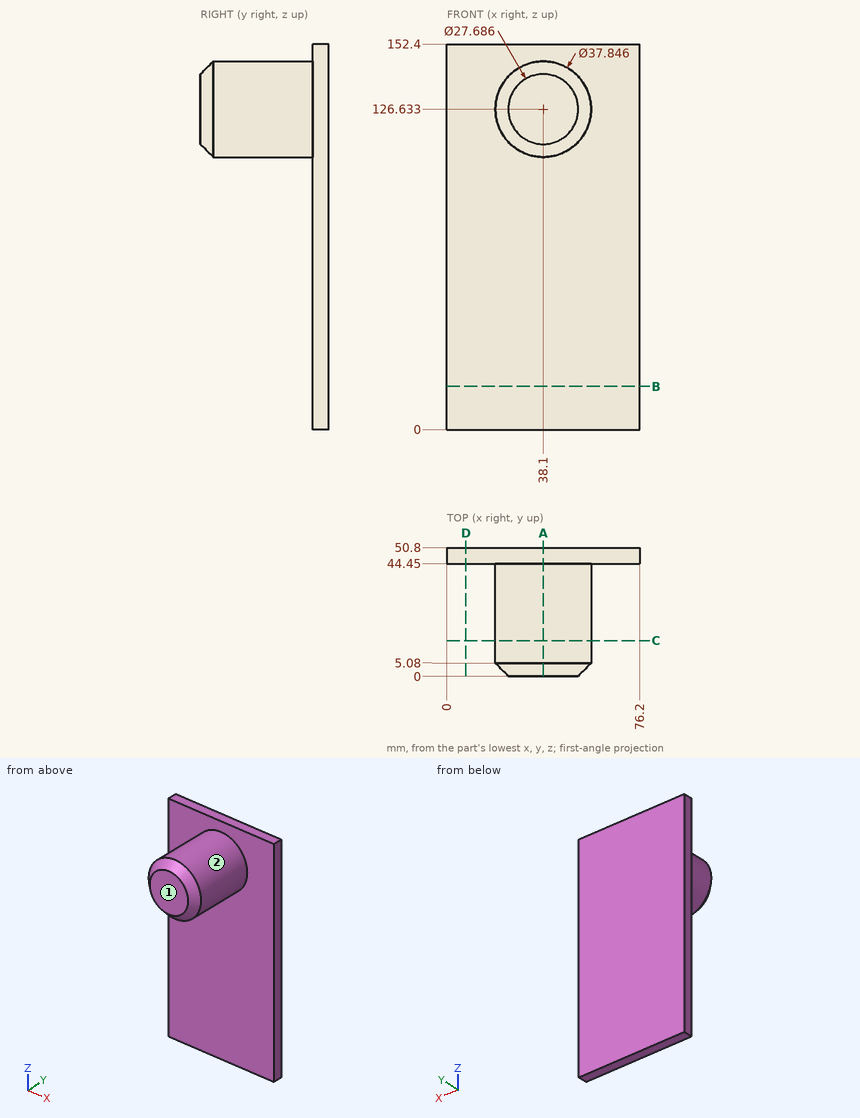
Here's the drawing with two shaded views (mm, measured from the low corner). I have some questions. A direction names the side the tool comes from. Give positions to 0.01 mm unless a question says otherwise; leave off trailing zeros. Order: outer loops, then holes, each group sorted by start corner. A loop starts at its lowest first (then second) coordinate and runs counter-clockwise, first axis right, second up. Notation, with made-up numbers: (89, 59.25) - (148, 59.25) arc R30 ccw to (148, 85.25) - close; hole circle Ø11 at (64.5, 37). An arc over 180 degrees is marked (long way). Use a Markdown table: item, result. Add a question column.
Q1. If we section it at D-D on x = 7.5: Write out the boundary of the cut face in (y, z).
Q2. I'm going to push flat-ended pins straight in: pin 1 (5 mm diameter, centred on y = 15, z = 120, fed in from -X); pin 2 (6 mm diameter, centred on y = 22, z = 111, fed in from -X); pin 3 (3 mm diameter, centred on x = 23.5, y = 5.5, fed in from -Z). Where does each tip first touch, or does it pass through?
Q3. If we section it at A-A on x = 38.1: Write out the boundary of the cut face in (y, z).
Q4. Please list where these lines run through material, in increasing order: line 1 along Y through (x, z) = (8, 125.5); line 2 along Z through (x, y) = (38, 34); line 3 along Z through (x, y) = (43, 14) (1 decimal).
Q5. If we section it at B-B on z = 17: Write out the boundary of the cut face in (x, y), plus the area to 3 significant figures.
Q6. On a 3-axis mill with a long thin cutter (end or side, diameter ignored), from which of +Z, -Z, +X, -X, +Y, -Y can I reach the whole of each face in a straight line? I mean the marked faces 1 and 2. Say none if no direction works.
Q7. If we section it at C-C on y = 14: Write out the boundary of the cut face in (x, z), plus the area to 4 significant figures.
Answers follow:
| question | item | result |
|---|---|---|
| 1 | outline | (44.45, 0) - (50.8, 0) - (50.8, 152.4) - (44.45, 152.4) - close |
| 2 | pin 1 | stops at x = 19.63 |
| 2 | pin 2 | stops at x = 24.01 |
| 2 | pin 3 | stops at z = 112.98 |
| 3 | outline | (0, 112.79) - (5.08, 107.71) - (44.45, 107.71) - (44.45, 0) - (50.8, 0) - (50.8, 152.4) - (44.45, 152.4) - (44.45, 145.56) - (5.08, 145.56) - (0, 140.48) - close |
| 4 | line 1 | y = 44.45 to 50.8 |
| 4 | line 2 | z = 107.71 to 145.56 |
| 4 | line 3 | z = 108.4 to 144.9 |
| 5 | outline | (0, 44.45) - (76.2, 44.45) - (76.2, 50.8) - (0, 50.8) - close |
| 5 | area | 484 mm^2 |
| 6 | face 1 | +Z, -Z, +X, -X, -Y |
| 6 | face 2 | -Y |
| 7 | outline | circle Ø37.85 at (38.1, 126.63) |
| 7 | area | 1,125 mm^2 |
